Read the model definition and answer for the solid it produces. Units are mm, in the model's axes. Coordinates: 2 decimals unless noted, no trailing zeros. Loops run counter-clockwise (first coordinate to the right, second up) from the corner with the lowest first, then second, coordinate; pieces in that order, holes last. Notation, with made-up numbers: (-9, 4) -> (41, 4) arc R17 ccw to (41, 10) -> close; hole circle Ø4 at (-3, 78). An arc over 180 degrees is marked (long way). Answer as CSV lines item,"result".
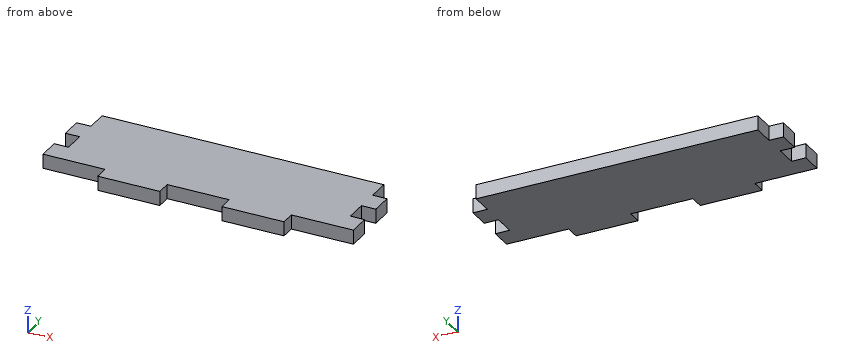
Autodesk Inventor part; units mm, degrees
ref_plane "YZ Plane" through (0, 0, 0) normal (1, 0, 0) x (0, 1, 0)
ref_plane "XZ Plane" through (0, 0, 0) normal (0, 1, 0) x (-1, 0, 0)
ref_plane "XY Plane" through (0, 0, 0) normal (0, 0, 1) x (1, 0, 0)
sketch "Sketch1" plane through (0, 0, 0) normal (0, 0, 1) x (1, 0, 0)
  line L0 (372, 110) -> (18, 110)
  line L1 (78, 0) -> (78, -18)
  line L2 (156, 0) -> (156, -18)
  line L3 (234, 0) -> (234, -18)
  line L4 (312, 0) -> (312, -18)
  line L5 (78, -18) -> (156, -18)
  line L6 (234, -18) -> (312, -18)
  line L7 (156, 0) -> (234, 0)
  line L8 (18, 27.5) -> (0, 27.5)
  line L9 (18, 55) -> (0, 55)
  line L10 (18, 55) -> (0, 55)
  line L11 (18, 82.5) -> (0, 82.5)
  line L12 (390, 82.5) -> (372, 82.5)
  line L13 (390, 55) -> (372, 55)
  line L14 (390, 27.5) -> (372, 27.5)
  line L15 (0, 0) -> (0, 27.5)
  line L16 (0, 55) -> (0, 82.5)
  line L17 (390, 0) -> (390, 27.5)
  line L18 (390, 55) -> (390, 82.5)
  line L19 (372, 27.5) -> (372, 55)
  line L20 (372, 82.5) -> (372, 110)
  line L21 (18, 110) -> (18, 82.5)
  line L22 (18, 55) -> (18, 27.5)
  line L23 (312, 0) -> (390, 0)
  line L24 (0, 0) -> (78, 0)
  dimension "d7" = 78
  dimension "d8" = 78
  dimension "d9" = 78
  dimension "d11" = 18
  dimension "d12" = 18
  dimension "d13" = 18
  dimension "d24" = 18
  dimension "d25" = 18
  dimension "d26" = 18
  dimension "d28" = 18
  dimension "d32" = 18
  dimension "d33" = 18
  dimension "d35" = 78
  dimension "d36" = 78
  dimension "d39" = 27.5
  dimension "d40" = 27.5
  dimension "d41" = 27.5
  dimension "d42" = 27.5
  dimension "d48" = 27.5
  dimension "d49" = 27.5
  dimension "d50" = 27.5
  dimension "d51" = 27.5
  dimension "d52" = 110
extrude "Extrusion3" add sketch "Sketch1" along normal blind 18
properties part number "cajon lat"
Q1. Find the intervals of material crossed by probe 1 along X at (y, z) = (94, 11.25); probe 2 along Y at (x, z) = (215, 16.5), in increasing order. Write a range as [from, to].
Results:
probe 1,"x = [18, 372]"
probe 2,"y = [0, 110]"
Q2. A cutting plane is placed at C-C, the plane x = 69.5. Write down the section's boundary in (y, z).
Results:
outline,"(0, 0) -> (110, 0) -> (110, 18) -> (0, 18) -> close"
Q3. A cutting plane is placed at A-A, the plane z = 9.5. Write down the section's boundary in (x, y).
Results:
outline,"(0, 0) -> (78, 0) -> (78, -18) -> (156, -18) -> (156, 0) -> (234, 0) -> (234, -18) -> (312, -18) -> (312, 0) -> (390, 0) -> (390, 27.5) -> (372, 27.5) -> (372, 55) -> (390, 55) -> (390, 82.5) -> (372, 82.5) -> (372, 110) -> (18, 110) -> (18, 82.5) -> (0, 82.5) -> (0, 55) -> (18, 55) -> (18, 27.5) -> (0, 27.5) -> close"
Q4. A cutting plane is placed at B-B, the plane y = 32. Write down the section's boundary in (x, z).
Results:
outline,"(18, 0) -> (372, 0) -> (372, 18) -> (18, 18) -> close"
Q5. Given pin 1 Ø5.5 at (y, z) = (-8.5, 12.5) entering from +X; pin 2 Ø9 at (x, z) = (342, 4.5) entering from -Y; pin 3 Ø9 at (x, z) = (381.5, 13) entering from +Y, each flat-ended and moving along its own axis, determine where each tip first touches the part or whether it passes through.
Results:
pin 1,"stops at x = 312"
pin 2,"stops at y = 0"
pin 3,"stops at y = 82.5"
